Build history of the part. All positions in model axes, mm. A direction names the side the tool comes from. Give positions to 0.01 mm unless a question says otherwise; leave off trailing zeros. Write each loop counter-clockwise with the first axis right and the second up, starting at its lowest first coordinate (ties: lowest second). Pieces come first, ordered by that corner, then holes. Notation, with made-up numbers: (-17, 45) -> (40, 45) arc R19 cw to (40, 74) -> close; hole circle Ø5 at (16.25, -9.5). An arc over 180 degrees is marked (long way). Put each result on its own line as item: value. Start each with the question number.
Item 1: Two-plate mould, pull along X, no slides. Class faces 1 (the flat face through (-57, 36, 3.81)), 2 (the cylindrical face through (1.127, -1.077, 1.556)), 3 (the flat face through (0, 35, 0)): pulls with the +X half, pulls with the -X half, needs draft (parallel to the pull), parting line crosses it, or undercut.
Item 2: Slice it at A-A, the plane z = 1.25. List the corners of the cut face in (x, y) (3 decimals), plus the area to 3 significant figures.
Item 3: Flat gauge pins, fed straight in: pin 1 Ø0.6 at (x, y) = (-52, 66.5) entering from +Z; pin 2 Ø2 at (x, y) = (-27, 6.5) entering from +Z; pin 3 Ø1 at (y, z) = (15.5, -3) entering from +X. Where does each tip first touch, or does it go through?
Item 4: Tool access for faces 4 (the cylindrical face through (-28.37, -1.08, -2.9)), 5 (the flat face through (-28, 70.688, 0)): list every direction of +Z, -Z, +X, -X, +Y, -Y with a clear straight run to the whole face (end or side of a thin tool).
Item 5: Drill centre lines: line 1 along X through (y, z) = (41.5, -0.25); line 2 along Y through (x, z) = (-14, 3.25); line 3 along Z through (x, y) = (-32, 21). Where is each one in solid material? Low to high.
Autodesk Inventor part; units mm, degrees
ref_plane "YZ Plane" through (0, 0, 0) normal (1, 0, 0) x (0, 1, 0)
ref_plane "XZ Plane" through (0, 0, 0) normal (0, 1, 0) x (-1, 0, 0)
ref_plane "XY Plane" through (0, 0, 0) normal (0, 0, 1) x (1, 0, 0)
sketch "Sketch1" plane through (0, 0, 0) normal (0, 0, 1) x (1, 0, 0)
  line L0 (0, 0) -> (0, 70.6882)
  line L1 (0, 70.6882) -> (-55.9816, 70.6882)
  line L2 (-55.9816, 70.6882) -> (-55.9816, 0)
  line L3 (-55.9816, 0) -> (0, 0)
  line L4 (-58.0136, 72.7202) -> (2.032, 72.7202)
  line L5 (2.032, 72.7202) -> (2.032, -2.032)
  line L6 (2.032, -2.032) -> (-58.0136, -2.032)
  line L7 (-58.0136, -2.032) -> (-58.0136, 72.7202)
  dimension "d0" = 70.6882
  dimension "d1" = 55.9816
  dimension "d2" = 70.6882
  dimension "d3" = 2.032
extrude "Extrusion1" add sketch "Sketch1" along normal mid plane 7.62
sketch "Sketch2" plane through (-55.9816, 0, 3.81) normal (1, 0, 0) x (0, 0, -1)
  line L0 (7.62, 72.7202) -> (0, 72.7202)
  line L1 (7.62, 72.7202) -> (6.858, 72.7202)
  line L2 (7.62, 70.6882) -> (0, 70.6882)
  line L3 (7.62, 70.6882) -> (6.7695, 70.6882)
  line L4 (6.7695, 70.6882) -> (6.7695, 0)
  line L5 (7.62, 0) -> (0, 0)
  line L6 (6.7695, 0) -> (7.62, 0)
  line L7 (7.62, 70.6882) -> (7.62, 0)
  line L8 (7.62, 0) -> (7.62, 70.6882)
  line L9 (7.62, 0) -> (7.62, 70.6882)
  line L10 (7.62, 70.6882) -> (6.8499, 70.6882)
  line L11 (0, 0) -> (7.62, 0)
  line L12 (6.7695, 0) -> (7.62, 0)
  line L13 (7.62, 0) -> (7.62, 70.6882)
  line L14 (6.6596, 0) -> (7.62, 0)
  line L15 (7.62, 72.7202) -> (7.62, -2.032)
  point P0 (3.81, 0)
  dimension "d6" = 0.762
  dimension "d7" = 70.6882
extrude "Extrusion2" add sketch "Sketch2" along normal blind 55.9816
sketch "Sketch3" plane through (-55.9816, 0, -2.9595) normal (0, 0, 1) x (1, 0, 0)
  line L0 (55.9816, 0) -> (0, 0)
  line L1 (55.9816, 70.6882) -> (55.9816, 0)
  circle A0 centre (51.9176, 4.064) radius 0.635
  line L2 (0, 0) -> (0, 70.6882)
  line L3 (0, 0) -> (0, 4.064)
  circle A1 centre (4.064, 4.064) radius 0.635
  line L4 (0, 70.6882) -> (55.9816, 70.6882)
  circle A2 centre (4.064, 66.6242) radius 0.635
  line L5 (55.9816, 70.6882) -> (55.9816, 66.6242)
  circle A3 centre (51.9176, 66.6242) radius 0.635
  dimension "d12" = 1.27
  dimension "d15" = 1.27
  dimension "d18" = 1.27
  dimension "d21" = 1.27
extrude "Extrusion3" add sketch "Sketch3" along normal blind 3.048 contours A0 | A1 | A2 | A3
fillet "Fillet1" radius 3.175 4 edges at (2.032, 72.7202, 0) (2.032, -2.032, 0) (-58.0136, 72.7202, 0) (-58.0136, -2.032, 0)
fillet "Fillet2" radius 3.175 8 edges at (1.1021, 71.7903, -3.81) (2.032, 35.3441, -3.81) (1.1021, -1.1021, -3.81) (-27.9908, -2.032, -3.81) (-57.0837, -1.1021, -3.81) (-58.0136, 35.3441, -3.81) (-57.0837, 71.7903, -3.81) (-27.9908, 72.7202, -3.81)
sketch "Sketch4" plane through (0, 0, 3.81) normal (0, 0, 1) x (1, 0, 0)
  line L0 (0, 0) -> (-55.9816, 0)
  line L1 (-54.8386, 1.143) -> (-1.143, 1.143)
  line L2 (-55.9816, 0) -> (-34.6456, 0)
  line L3 (-34.6456, 0) -> (-34.6456, 10.414)
  line L4 (-34.6456, 10.414) -> (-20.4216, 10.414)
  line L5 (-20.4216, 10.414) -> (-20.4216, 0)
  line L6 (0, 70.6882) -> (0, 0)
  line L7 (-20.4216, 0) -> (0, 0)
  dimension "d27" = 21.336
  dimension "d28" = 10.414
  dimension "d31" = 14.224
  dimension "d32" = 10.414
  dimension "d33" = 20.4216
properties part number "Box"
Values follow:
1. face 1: needs draft
1. face 2: pulls with the +X half
1. face 3: undercut
2. outline: (-58.014, 1.143) arc R3.175 ccw to (-54.839, -2.032) -> (-1.143, -2.032) arc R3.175 ccw to (2.032, 1.143) -> (2.032, 69.545) arc R3.175 ccw to (-1.143, 72.72) -> (-54.839, 72.72) arc R3.175 ccw to (-58.014, 69.545) -> close; hole (-55.982, 0) -> (0, 0) -> (0, 70.688) -> (-55.982, 70.688) -> close
2. area: 523 mm2
3. pin 1: z = 0.09
3. pin 2: z = -2.96
3. pin 3: x = 1.43
4. face 4: -Z, +X, -X, -Y
4. face 5: +Z
5. line 1: -58.01 to -55.98, 0 to 2.03
5. line 2: -2.03 to 0, 70.69 to 72.72
5. line 3: -3.81 to -2.96
